Geometry: final body of the model. Coordinates: model frame, mm. A direction names the side the tool comes from. Coordinates: 2 decimals unless noted, no trailing zeros. Order: outer loops, then holes, each group sorted by start corner. A loop starts at its lowest first (then second) coordinate and runs counter-clockwise, first axis right, second up. Notation, with made-up numbers: M -24,60.25 L 12,60.25 A18 ccw 12,65.25 Z; hole C 10.25,29.5 d7. An arc over 180 degrees is marked long. Use CSV: the item, a comma, the result in double quotes. Start each with the question number.
1. Section query D-D on y = 3.5. Return the cut outline in (x, z).
2. Material intervals for line 1 (Y direction, x = 11.45, z = 1.2); line 2 (Y direction, x = 11.75, z = 1); line 3 (Z direction, x = -0.5, y = 4.75), sorted ascending.
3. Set-up query: faces 4 (the cylindrical face through (-0.51, 5.33, 0.31)), 5 (the cylindrical face through (12.91, 4.07, 0.31)), 6 (the flat face through (11, -4.5, 1)), 7 (the flat face through (1.5, -4.5, 0.8)). Return all of +Z, -Z, +X, -X, +Y, -Y with unobstructed straight access to the full face (end or side cutting, diameter ignored); none if empty.
4. Section query C-C on x = 1.5. Return the cut outline in (y, z), and give its area (3 significant figures).
5. First-contact query: P1, Ø1.3, axis at x = 0.95, y = -6.1, coming from the +Z side; P2, Ø0.5, axis at y = 7.5, z = 1, coming from the +X side; P3, Ø0.5, axis at y = 2.5, z = 1, coming from the -X side. Flat tips, straight axial feed; report the tip coordinate or a pass-through.
6. Pull-direction query (X, two-part tool) for faces 1 (the cylindrical face through (-0.65, -6.06, 0.79)), 2 (the cylindrical face through (12.213, -5.86, 0.789)), 3 (the flat face through (11, 0, 1)); classes: pulls with the +X half, pulls with the -X half, needs draft (parallel to the pull), parting line crosses it, or undercut.
7. Section query A-A on y = -6.1. Return the cut outline in (x, z).
8. Section query B-B on z = 0.8. Return the cut outline in (x, y).
from build123d import *

# Parameters (mm, degrees)
F0_R     = 0.8
F1_DEPTH = 1.6
F2_W     = 3.14566
F2_H     = 3.226229
F2_R     = 0.8
F3_DEPTH = 1
F4_W     = 2.903376
F4_H     = 2.958158
F4_R     = 0.8
F5_DEPTH = 1


with BuildPart() as f1:
    # F0 (on Top) → F1 (new body)
    with BuildSketch(Plane.XY):
        with BuildLine():
            Line((0, 3.9), (0, 0))
            Line((0, 0), (1.95, 0))
            Line((1.95, 0), (1.95, -4.5))
            Line((1.95, -4.5), (0.95, -4.5))
            ThreePointArc((0.95, -4.5), (-0.65, -6.1), (0.95, -7.7))
            Line((0.95, -7.7), (11.45, -7.7))
            ThreePointArc((11.45, -7.7), (13.05, -6.1), (11.45, -4.5))
            Line((11.45, -4.5), (10.45, -4.5))
            Line((10.45, -4.5), (10.45, 0))
            Line((10.45, 0), (12.4, 0))
            Line((12.4, 0), (12.4, 3.9))
            Line((12.4, 3.9), (13.4, 3.9))
            Line((13.4, 3.9), (13.4, 5.5))
            Line((13.4, 5.5), (12.4, 5.5))
            Line((12.4, 5.5), (12.4, 9.4))
            Line((12.4, 9.4), (0, 9.4))
            Line((0, 9.4), (0, 5.5))
            Line((0, 5.5), (-1, 5.5))
            Line((-1, 5.5), (-1, 3.9))
            Line((-1, 3.9), (0, 3.9))
        make_face()
        with Locations((0.95, -6.1)):
            Circle(F0_R, mode=Mode.SUBTRACT)
        with Locations((11.45, -6.1)):
            Circle(F0_R, mode=Mode.SUBTRACT)
    extrude(amount=F1_DEPTH)

    # F2 (on face) → F3 (cut, through all)
    with BuildSketch(Plane(origin=(-1, 0, 0), x_dir=(0, -1, 0), z_dir=(-1, 0, 0))):
        with Locations((-4.643819, 0.893174)):
            Rectangle(F2_W, F2_H)
        with Locations((-4.7, 0.8)):
            Circle(F2_R, mode=Mode.SUBTRACT)
    extrude(amount=-F3_DEPTH, mode=Mode.SUBTRACT)

    # F4 (on face) → F5 (cut, through all)
    with BuildSketch(Plane.YZ.offset(13.4)):
        with Locations((4.745394, 0.737966)):
            Rectangle(F4_W, F4_H)
        with Locations((4.7, 0.8)):
            Circle(F4_R, mode=Mode.SUBTRACT)
    extrude(amount=-F5_DEPTH, mode=Mode.SUBTRACT)


solid = f1.part
Results list:
1,outline,"M 0,0 L 12.4,0 L 12.4,1.6 L 0,1.6 Z"
2,line 1,"y = -7.7 to -6.9, -5.3 to -4.5, 0 to 9.4"
2,line 2,"y = -7.67 to -6.84, -5.36 to -4.53, 0 to 9.4"
2,line 3,"z = 0 to 1.6"
3,face 4,"-X"
3,face 5,"+X"
3,face 6,"+Z, -Z, +X"
3,face 7,"+Z, -Z, -X"
4,outline,"M -7.7,0 L -6.68,0 L -6.68,1.6 L -7.7,1.6 Z; M -5.52,0 L -4.5,0 L -4.5,1.6 L -5.52,1.6 Z; M 0,0 L 9.4,0 L 9.4,1.6 L 0,1.6 Z"
4,area,"18.3 mm²"
5,P1,"passes through"
5,P2,"stops at x = 12.4"
5,P3,"stops at x = 0"
6,face 1,"pulls with the -X half"
6,face 2,"undercut"
6,face 3,"needs draft"
7,outline,"M -0.65,0 L 0.15,0 L 0.15,1.6 L -0.65,1.6 Z; M 1.75,0 L 10.65,0 L 10.65,1.6 L 1.75,1.6 Z; M 12.25,0 L 13.05,0 L 13.05,1.6 L 12.25,1.6 Z"
8,outline,"M -1,3.9 L 0,3.9 L 0,0 L 1.95,0 L 1.95,-4.5 L 0.95,-4.5 A1.6 ccw 0.95,-7.7 L 11.45,-7.7 A1.6 ccw 11.45,-4.5 L 10.45,-4.5 L 10.45,0 L 12.4,0 L 12.4,3.9 L 13.4,3.9 L 13.4,5.5 L 12.4,5.5 L 12.4,9.4 L 0,9.4 L 0,5.5 L -1,5.5 Z; hole C 0.95,-6.1 d1.6; hole C 11.45,-6.1 d1.6"
